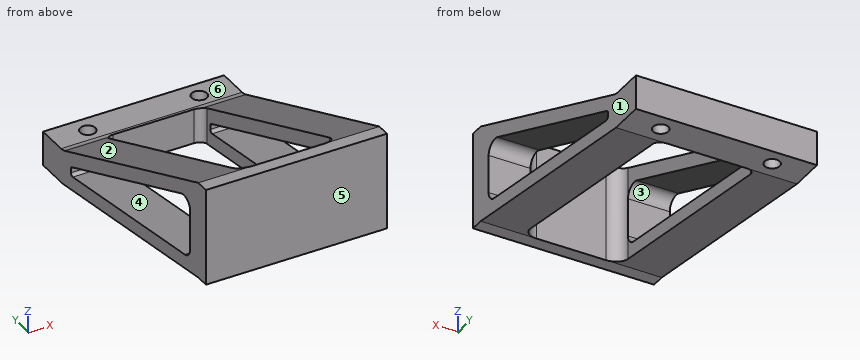
from build123d import *

# Parameters (mm, degrees)
BOSS_EXTRUDE1_DEPTH = 65
SKETCH2_W           = 35.00000000000001
SKETCH2_H           = 96.83750000000002
CUT_EXTRUDE1_DEPTH  = 130.59080671274705
FILLET1_R           = 5
CUT_EXTRUDE2_DEPTH  = 130.59080671274705
BOSS_EXTRUDE2_DEPTH = 35
SKETCH5_R           = 2.7500000000000084
SKETCH5_R_2         = 2.7499999999999956
CUT_EXTRUDE3_DEPTH  = 130.59080671274705
FILLET3_R           = 3


with BuildPart() as part:
    # Sketch1 → Boss-Extrude1 (new body)
    with BuildSketch(Plane(origin=(0, 0, 0), x_dir=(0, 0, -1), z_dir=(1, 0, 0))):
        with BuildLine():
            Line((47.39427375180004, 101.60000000000002), (47.39427375180004, 89.13544686995567))
            Line((47.39427375180004, 89.13544686995567), (35.000000000000014, 4.762500000000003))
            Line((35.000000000000014, 4.762500000000003), (35.000000000000014, 0))
            Line((35.000000000000014, 0), (0, 0))
            Line((0, 0), (0, 4.762500000000003))
            Line((0, 4.762500000000003), (34.54207855565439, 88.03155596440176))
            ThreePointArc((34.54207855565439, 88.03155596440176), (34.88440614395058, 89.15847126507197), (35.000000000000014, 90.3305481964365))
            Line((35.000000000000014, 90.3305481964365), (35.000000000000014, 101.60000000000002))
            Line((35.000000000000014, 101.60000000000002), (47.39427375180004, 101.60000000000002))
        make_face()
    extrude(amount=BOSS_EXTRUDE1_DEPTH)

    # Sketch2 → Cut-Extrude1 (cut, through all)
    with BuildSketch(Plane.XY):
        with Locations((32.50000000000001, 53.18125000000001)):
            Rectangle(SKETCH2_W, SKETCH2_H)
    extrude(amount=-CUT_EXTRUDE1_DEPTH, mode=Mode.SUBTRACT)

    # Fillet1
    fillet1_edges = [part.edges().sort_by_distance(p)[0] for p in [
        (50, 4.762500000000003, -17.500000000000007),
        (15, 4.762500000000003, -17.500000000000007),
    ]]
    fillet(fillet1_edges, radius=FILLET1_R)

    # Sketch3 → Cut-Extrude2 (cut, through all)
    with BuildSketch(Plane(origin=(65, 0, 0), x_dir=(0, 0, -1), z_dir=(1, 0, 0))):
        with BuildLine():
            Line((38.08312858614837, 83.51861224196143), (9.782341841456388, 15.295161488023126))
            ThreePointArc((9.782341841456388, 15.295161488023126), (10.15060285597038, 11.541086705731292), (13.477060878559312, 9.762500000000001))
            Line((13.477060878559312, 9.762500000000001), (27.225499843288624, 9.762500000000001))
            ThreePointArc((27.225499843288624, 9.762500000000001), (29.84032084558306, 10.735502952436189), (31.18302757021517, 13.181144437020006))
            Line((31.18302757021517, 13.181144437020006), (41.43787152872858, 82.99010797921063))
            ThreePointArc((41.43787152872858, 82.99010797921063), (41.20523885888791, 83.78915212052925), (40.44848959699694, 84.13544686995566))
            Line((40.44848959699694, 84.13544686995566), (39.006808345424105, 84.13544686995566))
            ThreePointArc((39.006808345424105, 84.13544686995566), (38.45145502185692, 83.96706137560288), (38.08312858614837, 83.51861224196143))
        make_face()
    extrude(amount=-CUT_EXTRUDE2_DEPTH, mode=Mode.SUBTRACT)

    # Sketch4 → Boss-Extrude2 (add)
    with BuildSketch(Plane(origin=(15, 0, 0), x_dir=(0, 0, -1), z_dir=(1, 0, 0))):
        with BuildLine():
            Line((47.39427375180004, 89.13544686995567), (47.39427375180004, 101.60000000000002))
            Line((47.39427375180004, 101.60000000000002), (35.000000000000014, 101.60000000000002))
            Line((35.000000000000014, 101.60000000000002), (35.000000000000014, 90.3305481964365))
            ThreePointArc((35.000000000000014, 90.3305481964365), (34.969867635356294, 89.72998145049917), (34.87977319455811, 89.13544686995567))
            Line((34.87977319455811, 89.13544686995567), (47.39427375180004, 89.13544686995567))
        make_face()
    extrude(amount=BOSS_EXTRUDE2_DEPTH)

    # Sketch5 → Cut-Extrude3 (cut, through all)
    with BuildSketch(Plane(origin=(0, 0, -47.39427375180004), x_dir=(-1, 0, 0), z_dir=(0, 0, -1))):
        with Locations((-52.50000000000002, 95.36772343497786)):
            Circle(SKETCH5_R)
        with Locations((-12.499999999999996, 95.36772343497786)):
            Circle(SKETCH5_R_2)
    extrude(amount=-CUT_EXTRUDE3_DEPTH, mode=Mode.SUBTRACT)

    # Fillet3
    fillet3_edges = [part.edges().sort_by_distance(p)[0] for p in [
        (15, 89.13544686995567, -41.13702347317908),
        (50, 89.13544686995567, -41.13702347317908),
    ]]
    fillet(fillet3_edges, radius=FILLET3_R)


solid = part.part
Here's how the part is built. I have some questions about the finished solid (model axes, mm). Face numbers are marked on the shaded views. A direction names the side the tool comes from. Coordinates: 2 decimals unless noted, no trailing zeros. Order: outer loops, then holes, each group sorted by start corner. A loop starts at its lowest first (then second) coordinate and runs counter-clockwise, first axis right, second up. Notation, with made-up numbers: (10.5, 0.25) -> (52.5, 0.25) arc R23 cw to (52.5, 32.25) -> close; hole circle Ø9 at (-0.75, -31). An arc over 180 degrees is marked (long way). Answer in a Markdown table with one row per item.
(1) I want a section at D-D on y = 48.5. List the corners of the cut face in (x, z) for me, then the cut area to 3 significant figures.
Answer key:
| item | result |
|---|---|
| outline | (0, -41.42) -> (15, -41.42) -> (15, -36.37) -> (0, -36.37) -> close; (0, -23.56) -> (15, -23.56) -> (15, -18.14) -> (0, -18.14) -> close; (50, -41.42) -> (65, -41.42) -> (65, -36.37) -> (50, -36.37) -> close; (50, -23.56) -> (65, -23.56) -> (65, -18.14) -> (50, -18.14) -> close |
| area | 314 mm^2 |
(2) I want a section at B-B on x = 29. List the corners of the cut face in (y, z) for me.
Answer key:
| item | result |
|---|---|
| outline | (0, -35) -> (4.76, -35) -> (4.76, 0) -> (0, 0) -> close; (89.14, -47.39) -> (101.6, -47.39) -> (101.6, -35) -> (90.33, -35) arc R6 cw to (89.14, -34.88) -> close |
(3) Please list where these lines run through material, in increasing order: probe 1 along X at (y, z) = (86, -43); probe 2 along Y at (x, z) = (41, -8.5); probe 3 along Z at (x, y) = (50, 92).
Answer key:
| item | result |
|---|---|
| probe 1 | 0 to 15, 50 to 65 |
| probe 2 | 0 to 4.76 |
| probe 3 | -47.39 to -35 |
(4) I want a section at C-C on z = -21. List the corners of the cut face in (x, y) for me, then the cut area to 3 significant figures.
Answer key:
| item | result |
|---|---|
| outline | (0, 0) -> (65, 0) -> (65, 9.76) -> (50, 9.76) arc R5 cw to (45, 4.76) -> (20, 4.76) arc R5 cw to (15, 9.76) -> (0, 9.76) -> close; (0, 42.34) -> (15, 42.34) -> (15, 55.39) -> (0, 55.39) -> close; (50, 42.34) -> (65, 42.34) -> (65, 55.39) -> (50, 55.39) -> close |
| area | 862 mm^2 |
(5) Thinking about a two-plate mould opening in Y: for the marked faces 1, 2 and 3, which applies, +Y half, -Y half, draft (parallel to the pull), parting line (faces both ways), or undercut?
Answer key:
| item | result |
|---|---|
| face 1 | draft |
| face 2 | +Y half |
| face 3 | undercut |
(6) Will these pins go through, and if not, where does the flat tip stop? pin 1 Ø3.5 at (x, y) = (19, 97.5) entering from +Z; pin 2 Ø15 at (x, z) = (60.5, -18) entering from +Y; pin 3 Ø12.5 at (x, z) = (33.5, -14.5) entering from +Y.
Answer key:
| item | result |
|---|---|
| pin 1 | z = -35 |
| pin 2 | y = 66.23 |
| pin 3 | y = 4.76 |
(7) I want a section at A-A on x = 52.5. List the corners of the cut face in (y, z) for me.
Answer key:
| item | result |
|---|---|
| outline | (0, -35) -> (4.76, -35) -> (89.14, -47.39) -> (92.62, -47.39) -> (92.62, -35) -> (90.33, -35) arc R6 cw to (88.03, -34.54) -> (4.76, 0) -> (0, 0) -> close; (98.12, -47.39) -> (101.6, -47.39) -> (101.6, -35) -> (98.12, -35) -> close; hole (9.76, -27.23) arc R4 ccw to (13.18, -31.18) -> (82.99, -41.44) arc R1 ccw to (84.14, -40.45) -> (84.14, -39.01) arc R1 ccw to (83.52, -38.08) -> (15.3, -9.78) arc R4 ccw to (9.76, -13.48) -> close |
(8) On a 3-axis mill with a long thin cutter (end or side, diameter ignored), from which of +Z, -Z, +X, -X, +Y, -Y can I reach the whole of each face in a straight line? I mean the marked faces 4, 5 and 6. Say none if no direction works.
Answer key:
| item | result |
|---|---|
| face 4 | +X, -X |
| face 5 | +Z, -Z, +X, -X, -Y |
| face 6 | +Z, +X, -X, +Y |
